Could you check a few things on this model? Use its own coordinates, in mm. Face numbers are marked on the shaded views. A direction names the side the tool comes from. Coordinates: 2 decimals unless noted, no trailing zeros. Write each loop counter-clockwise with the first axis right and the second up, starting at its lowest first coordinate (ties: lowest second). Pieces come first, ordered by that corner, then holes.
```python
from build123d import *

# Parameters (mm, degrees)
F1_DEPTH = 63.5
F2_DEPTH = 7.9375
F0_W     = 25.4
F0_H     = 19.05
F3_DEPTH = 25.4
F5_R     = 5.08


with BuildPart() as f1:
    # F0 (on Front) → F1 (new body, symmetric)
    with BuildSketch(Plane.XZ):
        Polygon((-41.275, -9.525), (41.275, -9.525), (41.275, 9.525), (22.225, 9.525), (-41.275, 9.525), align=None)
    extrude(amount=F1_DEPTH, both=True)

    # F0 (on Front) → F2 (join, symmetric)
    with BuildSketch(Plane.XZ):
        with BuildLine():
            add(Edge.make_bspline(
                [(-41.275, 9.525), (-33.9425614897, 49.4436582621), (6.8530607315, 60.3077269566), (55.0914084511, 61.8644772166)],
                knots=[0, 0, 0, 0, 109.9439298496, 109.9439298496, 109.9439298496, 109.9439298496], degree=3))
            Line((-41.275, 9.525), (22.225, 9.525))
            Line((22.225, 9.525), (22.225, 27.0002))
            ThreePointArc((22.225, 27.0002), (31.7368937864, 50.9570290384), (55.0914084511, 61.8644772166))
        make_face()
    extrude(amount=F2_DEPTH, both=True)

    # F0 (on Front) → F3 (join, symmetric)
    with BuildSketch(Plane.XZ):
        with BuildLine():
            Line((22.225, 9.525), (41.275, 9.525))
            Line((41.275, 9.525), (41.275, 27.0002))
            ThreePointArc((41.275, 27.0002), (45.9246798487, 38.2255201513), (57.15, 42.8752))
            Line((57.15, 42.8752), (60.325, 42.8752))
            Line((60.325, 42.8752), (60.325, 61.9252))
            Line((60.325, 61.9252), (57.15, 61.9252))
            add(Edge.make_bspline(
                [(55.0914084511, 61.8644772166), (55.7761308376, 61.8865746101), (56.4623528267, 61.9067967122), (57.15, 61.9252)],
                knots=[109.9439298496, 109.9439298496, 109.9439298496, 109.9439298496, 111.5045361635, 111.5045361635, 111.5045361635, 111.5045361635], degree=3))
            ThreePointArc((55.0914084511, 61.8644772166), (31.7368937864, 50.9570290384), (22.225, 27.0002))
            Line((22.225, 27.0002), (22.225, 9.525))
        make_face()
        with Locations((73.025, 52.4002)):
            Rectangle(F0_W, F0_H)
    extrude(amount=F3_DEPTH, both=True)

    # F0 (on Front) → F4 (revolve)
    with BuildSketch(Plane.XZ):
        Polygon((85.725, 61.9252), (85.725, 42.8752), (85.725, 38.1), (111.125, 38.1), (111.125, 66.675), (85.725, 66.675), align=None)
    revolve(axis=Axis((85.725, 0, 52.3875), (0, 0, 1)))

    # F5
    f5_edges = [f1.edges().sort_by_distance(p)[0] for p in [
        (-41.275, -63.5, 0),
        (41.275, -63.5, 0),
        (-41.275, 63.5, 0),
        (41.275, 63.5, 0),
    ]]
    fillet(f5_edges, radius=F5_R)


solid = f1.part
```
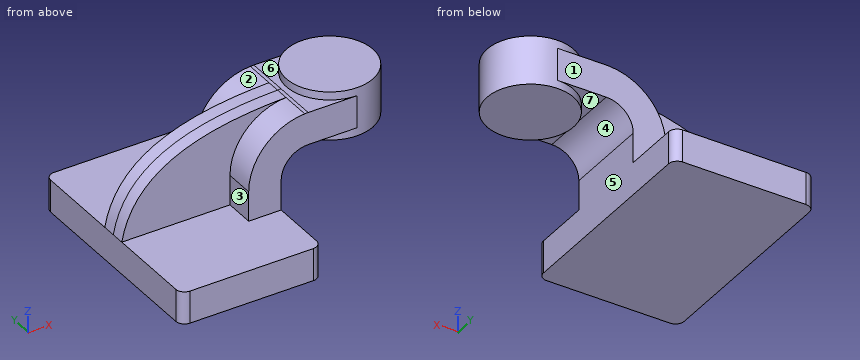
Item 1: I want a section at B-B, the plane y = 53.5. List the corners of the cut face in (x, z) for me (3 decimals).
Item 2: I want a section at A-A, the plane z = -0.5. List the corners of the cut face in (x, y) for me (3 decimals).
Item 3: Will these pins go through, and if not, where does the flat tip stop? pin 1 Ø8.5 at (y, z) = (-21, 18.5) entering from -X (3 decimals); pin 2 Ø2 at (x, y) = (9.5, -16.5) entering from +Z (3 decimals); pin 3 Ø5 at (x, z) = (27.5, 48.5) entering from +Y.
Item 4: I want a section at C-C, the plane x = 89. List the corners of the cut face in (y, z) for me (3 decimals).
Item 5: If I drill on line 1 along Z through (x, y) = (-28, 13.5) (3 decimals); line 2 along Z through (x, y) = (80, -2.5) (3 decimals); line 3 along X through (y, z) = (-15, -1) (3 decimals), over which ranges is the centre line in solid material (lowest first)?
Item 6: Which directions (+Z, -Z, +X, -X, +Y, -Y) give clear straight access to the entire face, cutting with the end or side of a thin tool? Please do the marked faces 1, 2 and 3.
Item 7: If we mould it in two halves opening along X, with no side actions, what happens to the marked faces 4, 5, 6 and 7? For each: released by +X, released by -X, zero draft, split by the parting line, or undercut.
Taken from the geometry:
1. outline: (-41.275, -9.525) - (41.275, -9.525) - (41.275, 9.525) - (-41.275, 9.525) - close
2. outline: (-41.275, -58.42) arc R5.08 ccw to (-36.195, -63.5) - (36.195, -63.5) arc R5.08 ccw to (41.275, -58.42) - (41.275, 58.42) arc R5.08 ccw to (36.195, 63.5) - (-36.195, 63.5) arc R5.08 ccw to (-41.275, 58.42) - close
3. pin 1: stops at x = 22.225
3. pin 2: stops at z = 9.525
3. pin 3: stops at y = 25.4
4. outline: (-25.188, 38.1) - (25.188, 38.1) - (25.188, 66.675) - (-25.188, 66.675) - close
5. line 1: z = -9.525 to 9.525
5. line 2: z = 38.1 to 66.675
5. line 3: x = -41.275 to 41.275
6. face 1: +Z, +X, -X, +Y
6. face 2: +Z, -X, +Y
6. face 3: +Z, -X, -Y
7. face 4: undercut
7. face 5: released by +X
7. face 6: zero draft
7. face 7: undercut
